Here's how the part is built. I have some questions about the finished solid (model axes, mm). Coordinates: 2 decimals unless noted, no trailing zeros. Write each loop counter-clockwise with the first axis right and the second up, starting at its lowest first coordinate (ties: lowest second). Pieces come first, ordered by that corner, then holes.
Item 1: If we section it at B-B (z = 0): Please give me the cut outline in (x, y), then the cut area to 3 significant figures.
Item 2: If I drill on line 1 (X direction, y = 0.15, z = -13.5); line 2 (X direction, y = 0.3, z = -11); line 3 (X direction, y = 0.25, z = 19), over which ranges is the centre line in solid material (lowest first)?
Item 3: I'm going to push a flat-ended pin straight in: pin 1 Ø1 at (x, z) = (19, -19.5) entering from -Y. Where does the tip first touch, or does it pass through?
Item 4: If we section it at A-A (x = 0): Please give me the cut outline in (y, z), then the cut area to 4 significant figures.
Item 5: If we section it at C-C (y = 0.2): Count the separate pieces of the cut face and the enclosed holes in it, then the cut area to 3 significant figures.
from build123d import *

# Parameters (mm, degrees)
SKETCH2_W               = 16.15
SKETCH2_H               = 0.35
CUT_EXTRUDE5_DEPTH      = 42.296519224
CIRPATTERN1_COUNT       = 12
CUT_EXTRUDE6_DEPTH      = 42.296519224
CUT_EXTRUDE6_DEPTH_BACK = 42.296519224
SKETCH5_R               = 1


with BuildPart() as part:
    # Sketch2 → Revolve2 (revolve)
    with BuildSketch(Plane.XY, mode=Mode.PRIVATE) as revolve2_sk:
        with Locations((21.125, 0.175)):
            Rectangle(SKETCH2_W, SKETCH2_H)
    revolve(revolve2_sk.sketch.rotate(Axis((0, 0, 0), (0, 1, 0)), 90), axis=Axis((0, 0, 0), (0, 1, 0)))

    # Sketch3 → Cut-Extrude5 (cut, symmetric)
    with BuildSketch(Plane(origin=(0, 0.35, 0), x_dir=(1, 0, 0), z_dir=(0, 1, 0))):
        with BuildLine():
            Line((-1.75, 19.287735518), (-1.75, 26.893121797))
            ThreePointArc((-1.75, 26.893121797), (-3.790597968, 26.682088881), (-5.809231237, 26.316446045))
            Line((-5.809231237, 26.316446045), (-6.29423199, 28.51355193))
            ThreePointArc((-6.29423199, 28.51355193), (-7.557516117, 28.205034128), (-8.805811164, 27.840576318))
            Line((-8.805811164, 27.840576318), (-8.127281194, 25.695326431))
            ThreePointArc((-8.127281194, 25.695326431), (-10.058290305, 25.002665781), (-11.931016442, 24.165126663))
            Line((-11.931016442, 24.165126663), (-8.128323302, 17.57866894))
            ThreePointArc((-8.128323302, 17.57866894), (-6.476196083, 16.129792255), (-4.283455194, 15.986072426))
            ThreePointArc((-4.283455194, 15.986072426), (-2.456345798, 17.206907895), (-1.75, 19.287735518))
        make_face()
    cut_extrude5 = extrude(amount=CUT_EXTRUDE5_DEPTH, both=True, mode=Mode.SUBTRACT)

    # CirPattern1: Cut-Extrude5 ×12 about axis
    cirpattern1_axis = Axis((0, 0, 0), (0, 1, 0))
    for i in range(1, CIRPATTERN1_COUNT):
        add(cut_extrude5.rotate(cirpattern1_axis, i * 360 / CIRPATTERN1_COUNT), mode=Mode.SUBTRACT)

    # Sketch5 → Cut-Extrude6 (cut, two sides: drawn at the far end of the back side and taken through both)
    with BuildSketch(Plane(origin=(0, 0.35, 0), x_dir=(1, 0, 0), z_dir=(0, 1, 0)).offset(-CUT_EXTRUDE6_DEPTH_BACK)):
        with Locations(Location((0, 15.765930428, 0), (0, 0, 270))):
            Circle(SKETCH5_R)
        with Locations(Location((0, -15.765930428, 0), (0, 0, 270))):
            Circle(SKETCH5_R)
    extrude(amount=CUT_EXTRUDE6_DEPTH + CUT_EXTRUDE6_DEPTH_BACK, mode=Mode.SUBTRACT)


solid = part.part
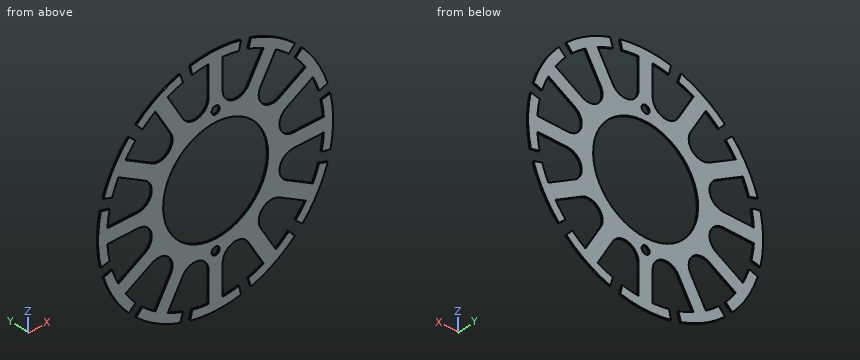
Answer list:
1. outline: (-29.2, 0) - (-13.05, 0) - (-13.05, 0.35) - (-29.2, 0.35) - close; (13.05, 0) - (29.2, 0) - (29.2, 0.35) - (13.05, 0.35) - close
1. area: 11.3 mm2
2. line 1: x = -25.89 to -19.88, -10.76 to 10.76, 19.88 to 25.89
2. line 2: x = -27.05 to -24.6, -22.55 to -15.52, -12.72 to -7.02, 7.02 to 12.72, 15.52 to 22.55, 24.6 to 27.05
2. line 3: x = -22.17 to -20.77, -12.99 to -8.95, -1.76 to 1.76, 8.95 to 12.99, 20.77 to 22.17
3. pin 1: passes through
4. outline: (0, -29.2) - (0.35, -29.2) - (0.35, -16.77) - (0, -16.77) - close; (0, -14.77) - (0.35, -14.77) - (0.35, -13.05) - (0, -13.05) - close; (0, 13.05) - (0.35, 13.05) - (0.35, 14.77) - (0, 14.77) - close; (0, 16.77) - (0.35, 16.77) - (0.35, 29.2) - (0, 29.2) - close
4. area: 9.905 mm2
5. separate pieces: 1
5. enclosed holes: 3
5. area: 1,120 mm2
